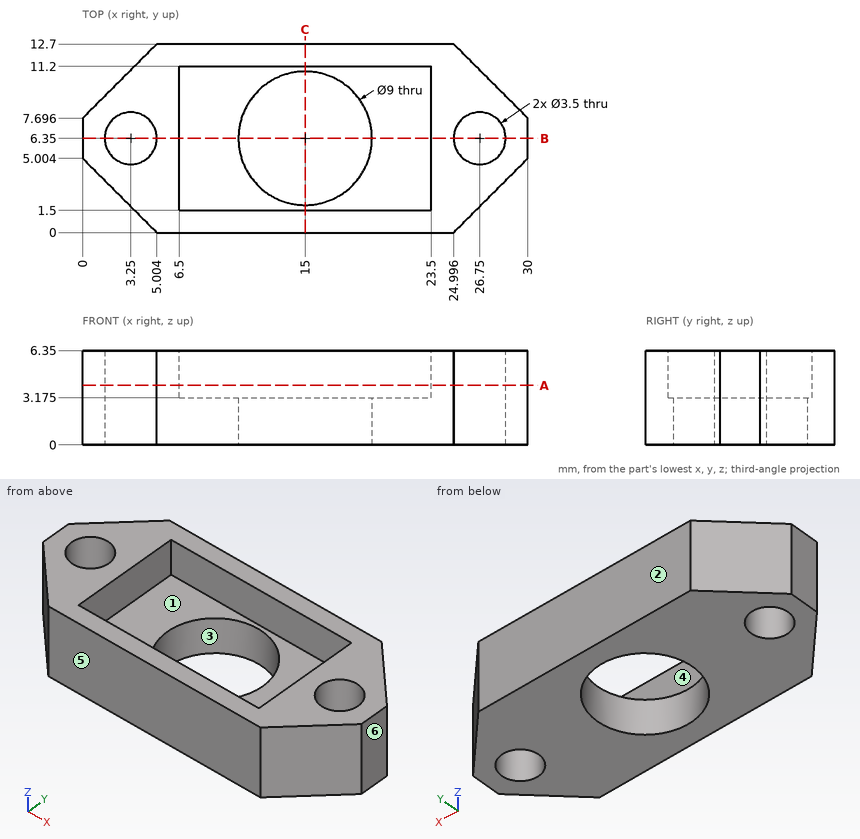
Geometry check sheet. Reference: drawing and pictorial views, mm from the part's lowest x, y, z. A direction names the side the tool comes from. Round coordinates to 2 decimals unless told otherwise and drop trailing zeros. Loops run counter-clockwise (first coordinate to the right, second up) from the corner with the lowest first, then second, coordinate; pieces in that order, holes last. Notation, with made-up numbers: (86.5, 64) - (137.5, 64) arc R6 ccw to (137.5, 70) - close; hole circle Ø1 at (38.5, 52). An arc over 180 degrees is marked (long way). One line per question, with ' | ' between items. Start each with the question number.
1. Scan lines: line 1 (X direction, y = 6.5, z = 4.25); line 2 (Y direction, x = 15, z = 1.9); line 3 (X direction, y = 6.75, z = 1.5). Record each from-to range of solid material in increasing order. Write a range as [from, to].
2. Depth check by flat-ended pin: pin 1 (1 mm diameter, centred on y = 8.5, z = 5, fed in from -X). Enter the tip coordinate at first touch or a pass-through.
3. Tool access check on the marked faces 1 and 2. Record the directions out of +Z, -Z, +X, -X, +Y, -Y that give a thin tool (end or side, any length) a straight path to the whole face; none if there is none.
4. Cross-section at B-B on y = 6.35. Record the cut outline in (x, z) (3 decimals), then the cut area to 3 significant figures.
5. Draft check along Y on the marked faces 3, 4, 5 and 6. Enter one of: released by +Y, released by -Y, zero draft, split by the parting line, or undercut.
6. Cross-section at A-A on z = 4. Record the cut outline in (x, y).
7. Cross-section at C-C on x = 15. Record the cut outline in (y, z) (3 decimals), then the cut area to 3 significant figures.
Taken from the geometry:
1) line 1: [0, 1.51], [4.99, 6.5], [23.5, 25.01], [28.49, 30] | line 2: [0, 1.85], [10.85, 12.7] | line 3: [0, 1.55], [4.95, 10.52], [19.48, 25.05], [28.45, 30]
2) pin 1: x = 0.3
3) face 1: +Z | face 2: +Z, -Z, +X, -X, +Y
4) outline: (0, 0) - (1.5, 0) - (1.5, 6.35) - (0, 6.35) - close; (5, 0) - (10.5, 0) - (10.5, 3.175) - (6.5, 3.175) - (6.5, 6.35) - (5, 6.35) - close; (19.5, 0) - (25, 0) - (25, 6.35) - (23.5, 6.35) - (23.5, 3.175) - (19.5, 3.175) - close; (28.5, 0) - (30, 0) - (30, 6.35) - (28.5, 6.35) - close | area: 63.5 mm²
5) face 3: undercut | face 4: undercut | face 5: released by -Y | face 6: zero draft
6) outline: (0, 5) - (5, 0) - (25, 0) - (30, 5) - (30, 7.7) - (25, 12.7) - (5, 12.7) - (0, 7.7) - close; hole circle Ø3.5 at (3.25, 6.35); hole (6.5, 1.5) - (23.5, 1.5) - (23.5, 11.2) - (6.5, 11.2) - close; hole circle Ø3.5 at (26.75, 6.35)
7) outline: (0, 0) - (1.85, 0) - (1.85, 3.175) - (1.5, 3.175) - (1.5, 6.35) - (0, 6.35) - close; (10.85, 0) - (12.7, 0) - (12.7, 6.35) - (11.2, 6.35) - (11.2, 3.175) - (10.85, 3.175) - close | area: 21.3 mm²
